Source: CAD feature listing. Evaluate the final solid. Frame: model axes, mm. A direction names the side the tool comes from. Round coordinates to 2 decimals unless told otherwise and drop trailing zeros. Loops run counter-clockwise (first coordinate to the right, second up) from the corner with the lowest first, then second, coordinate; pieces in that order, holes last. Notation, with made-up numbers: M 0.25,25.25 L 24.25,25.25 A24 ccw 24.25,60.25 Z; hole C -35,69.5 d8. An arc over 180 degrees is marked long. One line per item, written item: value.
from build123d import *

# Parameters (mm, degrees)
SKETCH1_R           = 75
BOSS_EXTRUDE1_DEPTH = 50
BOSS_EXTRUDE2_DEPTH = 50
BOSS_EXTRUDE3_DEPTH = 50
SKETCH4_R           = 25
CUT_EXTRUDE1_DEPTH  = 151


with BuildPart() as part:
    # Sketch1 → Boss-Extrude1 (new body)
    with BuildSketch(Plane(origin=(0, 0, 0), x_dir=(1, 0, 0), z_dir=(0, 1, 0))):
        Circle(SKETCH1_R)
    extrude(amount=BOSS_EXTRUDE1_DEPTH)

    # Sketch2 → Boss-Extrude2 (add)
    with BuildSketch(Plane(origin=(0, 50, 0), x_dir=(1, 0, 0), z_dir=(0, 1, 0))):
        with BuildLine():
            Line((-35, 0), (-35, -300))
            ThreePointArc((-35, -300), (0, -335), (35, -300))
            Line((35, -300), (35, 0))
            ThreePointArc((35, 0), (0, 35), (-35, 0))
        make_face()
    extrude(amount=BOSS_EXTRUDE2_DEPTH)

    # Sketch3 → Boss-Extrude3 (add)
    with BuildSketch(Plane(origin=(0, 100, 0), x_dir=(1, 0, 0), z_dir=(0, 1, 0))):
        with BuildLine():
            ThreePointArc((11.953887913, -332.895357784), (28.366317111, -320.502488959), (34.9848173, -301.03080477))
            ThreePointArc((34.9848173, -301.03080477), (34.996204119, -300.515458289), (35, -300))
            Line((35, -300), (35, -296.670788492))
            ThreePointArc((35, -296.670788492), (0.598184033, -264.595673491), (-35, -295.33761939))
            Line((-35, -295.33761939), (-35, -300))
            ThreePointArc((-35, -300), (-20.082503866, -328.665188617), (11.953887913, -332.895357784))
        make_face()
    extrude(amount=BOSS_EXTRUDE3_DEPTH)

    # Sketch4 → Cut-Extrude1 (cut, through all)
    with BuildSketch(Plane.XZ):
        Circle(SKETCH4_R)
    extrude(amount=-CUT_EXTRUDE1_DEPTH, mode=Mode.SUBTRACT)


solid = part.part
1. Section query A-A (z = -10.5). Return the cut outline in (x, y), and give its area (3 significant figures).
Report:
outline: M -74.26,0 L -22.69,0 L -22.69,100 L -33.39,100 L -33.39,50 L -74.26,50 Z; M 22.69,0 L 74.26,0 L 74.26,50 L 33.39,50 L 33.39,100 L 22.69,100 Z
area: 6,230 mm2
2. Ray query, line 1 (Z direction, x = 0, y = 54.5); line 2 (X direction, y = 89.5, z = 278); line 3 (Y direction, x = -66.5, z = 14). Return the intervals inside material, ascending. Write a range as [from, to].
Report:
line 1: z = [-35, -25], [25, 335]
line 2: x = [-35, 35]
line 3: y = [0, 50]
3. Reachability of faces 4 (the face through (-9.764, 24.65, -74.362)), 5 (the face through (-35, 77, 148)), 6 (the face through (0.77, 74.65, -34.99)), 7 (the face through (-18, 0, -18)) from +Z, -Z, +X, -X, +Y, -Y: full face, straight path, thin tool, end or side. Return the list, or none.
Report:
face 4: -Y
face 5: +Z, -Z, -X, +Y
face 6: -Z, +Y
face 7: +Z, -Z, +X, -X, -Y
4. Pull-direction query (Z, two-part tool) for faces 1 (the face through (35, 77, 152)), 2 (the face through (23.846, 49.3, 7.509)), 3 (the face through (1.319, 124.65, 264.617)); classes: released by +Z, released by -Z, zero draft, split by the parting line, or undercut.
Report:
face 1: zero draft
face 2: undercut
face 3: released by -Z
5. Section query C-C (x = -5.5). Return the cut outline in (y, z).
Report:
outline: M 0,-74.8 L 50,-74.8 L 50,-34.57 L 100,-34.57 L 100,-24.39 L 0,-24.39 Z; M 0,24.39 L 100,24.39 L 100,265.01 L 150,265.01 L 150,334.57 L 50,334.57 L 50,74.8 L 0,74.8 Z
6. Section query B-B (y = 74.5). Return the cut outline in (x, z).
Report:
outline: M -35,0 A35 ccw 35,0 L 35,300 A35 ccw -35,300 Z; hole C 0,0 d50
7. Pin query (flat end, axial travel): pin 1 (5 mm diameter, centred on x = 4, z = 155, fed in from +Y); pin 2 (10 mm diameter, centred on x = -47, y = 33.5, fed in from +Z); pin 3 (2 mm diameter, centred on y = 92.5, z = 203.5, fed in from +X); pin 4 (1 mm diameter, centred on y = 49, z = 91, fed in from -X). Return the tip coordinate at first contact, or that it passes through.
Report:
pin 1: stops at y = 100
pin 2: stops at z = 62.14
pin 3: stops at x = 35
pin 4: passes through
8. Section query D-D (z = 285). Return the cut outline in (x, y).
Report:
outline: M -35,50 L 35,50 L 35,100 L 31.88,100 L 31.88,150 L -32.02,150 L -32.02,100 L -35,100 Z
